The model under review builds one solid part; all positions refer to its coordinate system, in mm. A direction names the side the tool comes from. Coordinates: 2 decimals unless noted, no trailing zeros. Write each loop counter-clockwise with the first axis right and the second up, starting at its lowest first coordinate (ties: lowest second). Pieces come first, ordered by that corner, then holes. Notation, with made-up numbers: (31.25, 40) - (55.25, 40) arc R23 cw to (55.25, 63) - close; hole circle Ø7 at (72, 30). An arc over 180 degrees is marked (long way). Put each result on its own line as item: value. Start each with the question number.
Item 1: For pin 1 (3 mm diameter, centred on y = 0, z = 8, fed in from +X); pin 2 (3 mm diameter, centred on x = 9.5, z = 9, fed in from +Y); pin 3 (8 mm diameter, centred on x = -29.5, z = 6, fed in from +Y), all flat-tipped, find the tip position at first contact; note any pin that passes through.
Item 2: Mouldability with a two-part tool opening along X and no side actions: class faces 1 (the face through (52, 0, 8)), 2 (the face through (40.147, -0.209, 9.498)), 3 (the face through (0, 16, 0)), 4 (the face through (-52, 0, 8)) as pulls with the +X half, pulls with the -X half, needs draft (parallel to the pull), parting line crosses it, or undercut.
Item 3: Machinability: for faces 5 (the face through (0, 0, 17)), 6 (the face through (-55, 0, 10)), 7 (the face through (35, 0, 10)), 8 (the face through (50.99, -0.16, 7.5)), which of the approach directions +Z, -Z, +X, -X, +Y, -Y give a long, thin tool a straight path to every point of the face, cutting with its end or side? Answer none if there is none.
Item 4: To check wall thickness, follow L1, parallel to X at y = 12, z = 3.5; L2, parallel to X at y = -10, z = 8.5; L3, parallel to Y at x = -46.5, z = 7.25. State the ranges of each line that lie inside material, in increasing order. Write a range as [from, to].
Item 5: Consider section A-A on x = -31. Give the boundary of the cut face in (y, z).
```python
from build123d import *

# Parameters (mm, degrees)
REVOLUTION_ANGLE = -180
SKETCH001_W      = 34
SKETCH001_H      = 1
PAD_DEPTH        = 1
SKETCH002_W      = 36
SKETCH002_H      = 1.5
POCKET_DEPTH     = 1
SKETCH003_R      = 4
PAD001_DEPTH     = 8


with BuildPart() as part:
    # Sketch → Revolution (revolve)
    with BuildSketch(Plane.XY):
        with BuildLine():
            Line((-35, -17), (35, -17))
            ThreePointArc((35, -17), (46.543396, -15.207817), (57, -10))
            Line((57, -10), (52, -10))
            Line((52, -10), (52, -7.5))
            Line((52, -7.5), (50, -7.5))
            Line((50, -7.5), (50, -11.758585))
            ThreePointArc((48, -12.600664), (49.00633, -12.194658), (50, -11.758585))
            Line((48, -9.5), (48, -12.600664))
            Line((35, -9.5), (48, -9.5))
            Line((35, -14), (35, -9.5))
            Line((35, -14), (-35, -14))
            Line((-35, -14), (-35, -9.5))
            Line((-35, -9.5), (-48, -9.5))
            Line((-48, -9.5), (-48, -12.600664))
            ThreePointArc((-50, -11.758585), (-49.00633, -12.194658), (-48, -12.600664))
            Line((-50, -11.758585), (-50, -7.5))
            Line((-50, -7.5), (-52, -7.5))
            Line((-52, -7.5), (-52, -10))
            Line((-52, -10), (-57, -10))
            ThreePointArc((-57, -10), (-46.543396, -15.207817), (-35, -17))
        make_face()
    revolve(axis=Axis((0, 0, 0), (1, 0, 0)), revolution_arc=REVOLUTION_ANGLE)

    # Sketch001 → Pad (new body)
    with BuildSketch(Plane.XY):
        with Locations((18, 14.5)):
            Rectangle(SKETCH001_W, SKETCH001_H)
    pad = extrude(amount=-PAD_DEPTH)

    # Mirrored: Pad across XZ
    add(pad.mirror(Plane.XZ))

    # Sketch002 → Pocket (cut)
    with BuildSketch(Plane.XY):
        with Locations((-17, 14.75)):
            Rectangle(SKETCH002_W, SKETCH002_H)
    pocket = extrude(amount=POCKET_DEPTH, mode=Mode.SUBTRACT)

    # Mirrored001: Pocket across XZ
    add(pocket.mirror(Plane.XZ), mode=Mode.SUBTRACT)

    # Sketch003 → Pad001 (join)
    with BuildSketch(Plane.XY):
        with Locations((43, -8)):
            Circle(SKETCH003_R)
        with Locations((-43, -8)):
            Circle(SKETCH003_R)
        with Locations((-43, 8)):
            Circle(SKETCH003_R)
        with Locations((43, 8)):
            Circle(SKETCH003_R)
    extrude(amount=PAD001_DEPTH)


solid = part.part
```
Report:
1. pin 1: x = 52
1. pin 2: y = 15.26
1. pin 3: y = 16.88
2. face 1: pulls with the +X half
2. face 2: undercut
2. face 3: needs draft
2. face 4: pulls with the -X half
3. face 5: +Z, +X, -X
3. face 6: -Z, -X
3. face 7: -Z
3. face 8: -Z, +X
4. L1: [-52.96, -48.26], [-48, -35], [35, 48], [48.26, 52.96]
4. L2: [-51.74, -35], [35, 51.74]
4. L3: [-13.38, -6.06], [6.06, 13.38]
5. outline: (-17, 0) - (-15.5, 0) - (-15.5, 1) - (-14, 1) - (-14, 0) arc R14 cw to (14, 0) - (14, 1) - (15.5, 1) - (15.5, 0) - (17, 0) arc R17 ccw to start
